Design review of the part built by this model. Coordinates are the model's own, in mm. A direction names the side the tool comes from. Coordinates: 2 decimals unless noted, no trailing zeros. Loops run counter-clockwise (first coordinate to the right, second up) from the corner with the lowest first, then second, coordinate; pieces in that order, holes last. Notation, with made-up numbers: M 14.25,-8 L 47.25,-8 A25 cw 47.25,14 Z; hole C 6,22.5 d3. An arc over 180 degrees is marked long. Put each result on its own line as item: value. Start each with the question number.
(1) Take a section at A-A, the plane y = -8. Give the boundary of the cut face in (x, z).
(2) Take a section at C-C, the plane z = 33.5. Give the boundary of the cut face in (x, y), then the cut area to 3 significant figures.
(3) Take a section at B-B, the plane x = 28.5. Give the boundary of the cut face in (y, z), then the cut area to 3 significant figures.
(4) For faces 1 (the flat face through (32, -6, 10.454)), 2 (the flat face through (19, -6, 0)), list the 3-axis set-ups (+Z, -Z, +X, -X, +Y, -Y) from which the entire face can be reached by the end or side of a thin tool; tool diameter is ignored.
(5) Clearance check with flat-ended pins moving along their axes: pin 1 (8 mm diameter, centred on y = -14.5, z = 26.5, fed in from +X); pin 2 (1 mm diameter, centred on x = 31.5, y = -10.5, fed in from +Z); pin 3 (14 mm diameter, centred on x = 31.5, y = -10, fed in from +Z). State where each tip first meets the part, or that it passes through.
(6) For probe 1 along Z at (x, y) = (34, 5.5); probe 2 along X at (y, z) = (0.25, 25); probe 3 along Z at (x, y) = (15, -12.5), list the stretches that pass through material, from the lowest coordinate up. Write a range as [from, to].
```python
from build123d import *

# Parameters (mm, degrees)
F0_W     = 25.4
F0_H     = 38.1
F1_DEPTH = 38.1
F3_DEPTH = 25.4


with BuildPart() as f1:
    # F0 (on Right) → F1 (new body)
    with BuildSketch(Plane.YZ):
        with Locations((-5.703593, 19.05)):
            Rectangle(F0_W, F0_H)
    extrude(amount=F1_DEPTH)

    # F2 (on face) → F3 (cut)
    with BuildSketch(Plane.XZ.offset(18.403593)):
        Polygon((38.1, 38.1), (12.7, 38.1), (25.4, 10.454088), (38.1, 10.454088), align=None)
    extrude(amount=-F3_DEPTH, mode=Mode.SUBTRACT)


solid = f1.part
```
Computed values:
1. outline: M 0,0 L 38.1,0 L 38.1,10.45 L 25.4,10.45 L 12.7,38.1 L 0,38.1 Z
2. outline: M 0,-18.4 L 14.81,-18.4 L 14.81,7 L 0,7 Z
2. area: 376 mm^2
3. outline: M -18.4,0 L 7,0 L 7,10.45 L -18.4,10.45 Z
3. area: 266 mm^2
4. face 1: +Z, +X, +Y, -Y
4. face 2: -Z, +X, -X, +Y, -Y
5. pin 1: stops at x = 19.87
5. pin 2: stops at z = 10.45
5. pin 3: stops at z = 12.41
6. probe 1: z = [0, 10.45]
6. probe 2: x = [0, 18.72]
6. probe 3: z = [0, 33.09]
